CAD build for the part. Positions are in the model's coordinates, mm. A direction names the side the tool comes from. Give positions to 0.01 mm unless a question says otherwise; leave off trailing zeros. Loops run counter-clockwise (first coordinate to the right, second up) from the corner with the lowest first, then second, coordinate; pieces in that order, holes last. Notation, with made-up numbers: (-14.75, 71) -> (5.25, 71) arc R11 cw to (5.25, 76) -> close; hole circle Ø4 at (54.5, 11.25). An arc over 180 degrees is marked (long way). Use one line per item in the form item = value.
```python
from build123d import *

# Parameters (mm, degrees)
SKETCH1_R               = 69
BOSS_EXTRUDE1_DEPTH     = 50
SKETCH2_W               = 125
SKETCH2_H               = 125
BOSS_EXTRUDE2_DEPTH     = 3
SKETCH3_R               = 2.75
CUT_EXTRUDE1_DEPTH      = 3
SKETCH4_R               = 66
CUT_EXTRUDE2_DEPTH      = 110.644881321
FILLET1_R               = 10
CUT_EXTRUDE3_DEPTH      = 110.644881321
BOSS_EXTRUDE4_DEPTH     = 50
CIRPATTERN2_COUNT       = 4
BOSS_EXTRUDE5_DEPTH     = 50
CUT_EXTRUDE4_DEPTH      = 20
CUT_EXTRUDE4_DEPTH_BACK = 20
SKETCH10_R              = 66
SKETCH11_R              = 15
BOSS_EXTRUDE6_DEPTH     = 50
SKETCH14_R              = 12
CUT_EXTRUDE6_DEPTH      = 110.644881494


with BuildPart() as part:
    # Sketch1 → Boss-Extrude1 (new body)
    with BuildSketch(Plane(origin=(0, 0, 0), x_dir=(1, 0, 0), z_dir=(0, 1, 0))):
        with Locations(Location((0, 0, 0), (0, 0, 270))):
            Circle(SKETCH1_R)
    extrude(amount=BOSS_EXTRUDE1_DEPTH)

    # Sketch2 → Boss-Extrude2 (add)
    with BuildSketch(Plane(origin=(0, 50, 0), x_dir=(1, 0, 0), z_dir=(0, 1, 0))):
        Rectangle(SKETCH2_W, SKETCH2_H)
    extrude(amount=-BOSS_EXTRUDE2_DEPTH)

    # Sketch3 → Cut-Extrude1 (cut)
    with BuildSketch(Plane(origin=(0, 50, 0), x_dir=(1, 0, 0), z_dir=(0, 1, 0))):
        with Locations(Location((55, 55, 0), (0, 0, 270))):
            Circle(SKETCH3_R)
        with Locations(Location((-55, 55, 0), (0, 0, 270))):
            Circle(SKETCH3_R)
        with Locations(Location((-55, -55, 0), (0, 0, 270))):
            Circle(SKETCH3_R)
        with Locations(Location((55, -55, 0), (0, 0, 270))):
            Circle(SKETCH3_R)
    extrude(amount=-CUT_EXTRUDE1_DEPTH, mode=Mode.SUBTRACT)

    # Sketch4 → Cut-Extrude2 (cut, through all)
    with BuildSketch(Plane.XZ):
        with Locations(Location((0, 0, 0), (0, 0, 270))):
            Circle(SKETCH4_R)
    extrude(amount=-CUT_EXTRUDE2_DEPTH, mode=Mode.SUBTRACT)

    # Fillet1
    fillet1_edges = [part.edges().sort_by_distance(p)[0] for p in [
        (-62.5, 48.5, 62.5),
        (-62.5, 48.5, -62.5),
        (62.5, 48.5, -62.5),
        (62.5, 48.5, 62.5),
    ]]
    fillet(fillet1_edges, radius=FILLET1_R)

    # Sketch6 → Cut-Extrude3 (cut, through all)
    with BuildSketch(Plane(origin=(0, 0, 0), x_dir=(0, 0, -1), z_dir=(1, 0, 0))):
        with BuildLine():
            Line((-8, 0), (-8, 12))
            ThreePointArc((-8, 12), (0, 20), (8, 12))
            Line((8, 12), (8, 0))
            ThreePointArc((8, 0), (0, -8), (-8, 0))
        make_face()
    extrude(amount=CUT_EXTRUDE3_DEPTH, mode=Mode.SUBTRACT)

    # Sketch8 → Boss-Extrude4 (add)
    with BuildSketch(Plane(origin=(0, 50, 0), x_dir=(1, 0, 0), z_dir=(0, 1, 0))):
        Polygon((41.790010768, 54.659354186), (33.870414819, 46.739758236), (46.739758236, 33.870414819), (54.659354186, 41.790010768), align=None)
        Polygon((41.790010768, 50.416713499), (50.416713499, 41.790010768), (46.739758236, 38.113055506), (38.113055506, 46.739758236), align=None, mode=Mode.SUBTRACT)
    boss_extrude4 = extrude(amount=-BOSS_EXTRUDE4_DEPTH)

    # CirPattern2: Boss-Extrude4 ×4 about axis
    cirpattern2_axis = Axis((0, 0, 0), (0, 1, 0))
    for i in range(1, CIRPATTERN2_COUNT):
        add(boss_extrude4.rotate(cirpattern2_axis, i * 360 / CIRPATTERN2_COUNT))

    # Sketch9 → Boss-Extrude5 (add)
    with BuildSketch(Plane(origin=(0, 50, 0), x_dir=(1, 0, 0), z_dir=(0, 1, 0))):
        Polygon((46.739758236, 33.870414819), (33.870414819, 46.739758236), (0, 8), (-33.870414819, 46.739758236), (-46.739758236, 33.870414819), (-8, 0), (-46.739758236, -33.870414819), (-33.870414819, -46.739758236), (0, -8), (33.870414819, -46.739758236), (46.739758236, -33.870414819), (8, 0), align=None)
    extrude(amount=-BOSS_EXTRUDE5_DEPTH)

    # Sketch10 → Cut-Extrude4 (cut, two sides: drawn at the far end of the back side and taken through both)
    with BuildSketch(Plane(origin=(0, 25, 0), x_dir=(1, 0, 0), z_dir=(0, 1, 0)).offset(-CUT_EXTRUDE4_DEPTH_BACK)):
        with Locations(Location((0, 0, 0), (0, 0, 52.925119379))):
            Circle(SKETCH10_R)
    extrude(amount=CUT_EXTRUDE4_DEPTH + CUT_EXTRUDE4_DEPTH_BACK, mode=Mode.SUBTRACT)

    # Sketch11 → Boss-Extrude6 (add)
    with BuildSketch(Plane.XZ):
        with Locations(Location((0, 0, 0), (0, 0, 290.612180744))):
            Circle(SKETCH11_R)
    extrude(amount=-BOSS_EXTRUDE6_DEPTH)

    # Sketch14 → Cut-Extrude6 (cut, through all)
    with BuildSketch(Plane(origin=(0, 50, 0), x_dir=(1, 0, 0), z_dir=(0, 1, 0))):
        with Locations(Location((0, 0, 0), (0, 0, 270))):
            Circle(SKETCH14_R)
    extrude(amount=-CUT_EXTRUDE6_DEPTH, mode=Mode.SUBTRACT)


solid = part.part
```
1. Cut at B-B, the plane z = -18. Write the cut outline in (x, y), then the cut area to 3 significant figures.
Result sheet:
outline = (-66.61, 0) -> (-63.5, 0) -> (-63.5, 50) -> (-66.61, 50) -> close; (-28.59, 0) -> (-8.74, 0) -> (-8.74, 5) -> (-28.59, 5) -> close; (-28.59, 45) -> (-8.74, 45) -> (-8.74, 50) -> (-28.59, 50) -> close; (8.74, 0) -> (28.59, 0) -> (28.59, 5) -> (8.74, 5) -> close; (8.74, 45) -> (28.59, 45) -> (28.59, 50) -> (8.74, 50) -> close; (63.5, 0) -> (66.61, 0) -> (66.61, 50) -> (63.5, 50) -> close
area = 708 mm^2
2. Tool access for faces 1 (the flat face through (42.487, 2.535, -42.366)), 2 (the flat face through (-28, 45, 29)), 3 (the flat face through (-52, 47, 53)): list every direction of +Z, -Z, +X, -X, +Y, -Y with a clear straight run to the whole face (end or side of a thin tool).
Result sheet:
face_1 = +Y, -Y
face_2 = none
face_3 = +Z, -X, -Y
3. Cut at A-A, the plane y = 9.5. Write the cut outline in (x, z), then the cut area to 3 significant figures.
Result sheet:
outline = circle Ø30 at (0, 0); (65.51, -8) arc R66 cw (long way) to (65.51, 8) -> (68.53, 8) arc R69 ccw (long way) to (68.53, -8) -> close; hole circle Ø24 at (0, 0)
area = 1,480 mm^2
4. Drop flat-ended pins along their axis: P1, Ø1.5, axis at y = 48, z = 44, coming from the +X side; P2, Ø3.5, axis at x = 43.5, y = 48, coming from the +Z side; P3, Ø2.5, axis at x = 44.5, y = 48, coming from the -Z side. Give the stop position or say it passes through.
Result sheet:
P1 = 62.5
P2 = 62.5
P3 = -62.5
5. Mould opens along X. For faces 4 (the cylindrical face through (3.034, 24.65, -68.933)), 5 (the flat face through (42.366, 2.535, 42.487)), 6 (the flat face through (52, 47, -52)) say: pulls with the +X half, pulls with the -X half, needs draft (parallel to the pull), parting line crosses it, or undercut.
Result sheet:
face_4 = parting line crosses it
face_5 = undercut
face_6 = needs draft
6. Cut at C-C, the plane x = 55. Write the cut outline in (y, z), then the cut area to 3 significant figures.
Result sheet:
outline = (0, -41.67) -> (47, -41.67) -> (47, -52.25) -> (50, -52.25) -> (50, -36.48) -> (0, -36.48) -> close; (0, 36.48) -> (50, 36.48) -> (50, 52.25) -> (47, 52.25) -> (47, 41.67) -> (0, 41.67) -> close; (47, -62.18) -> (50, -62.18) -> (50, -57.75) -> (47, -57.75) -> close; (47, 57.75) -> (50, 57.75) -> (50, 62.18) -> (47, 62.18) -> close
area = 608 mm^2
7. Cut at D-D, the plane y = 43. Write the cut outline in (x, z).
Result sheet:
outline = circle Ø138 at (0, 0); circle Ø30 at (0, 0); hole circle Ø132 at (0, 0); hole circle Ø24 at (0, 0)
8. Drill centre lines: line 1 (Y direction, x = -21.5, z = -31.5); line 2 (X direction, y = 48, z = -55); line 3 (X direction, y = 3, z = 5.5). Where is each one in solid material? Low to high.
Result sheet:
line_1 = 0 to 5, 45 to 50
line_2 = -62.18 to -57.75, -52.25 to -36.48, 36.48 to 52.25, 57.75 to 62.18
line_3 = -68.78 to -65.77, -14.29 to -10.67, 10.67 to 14.29
